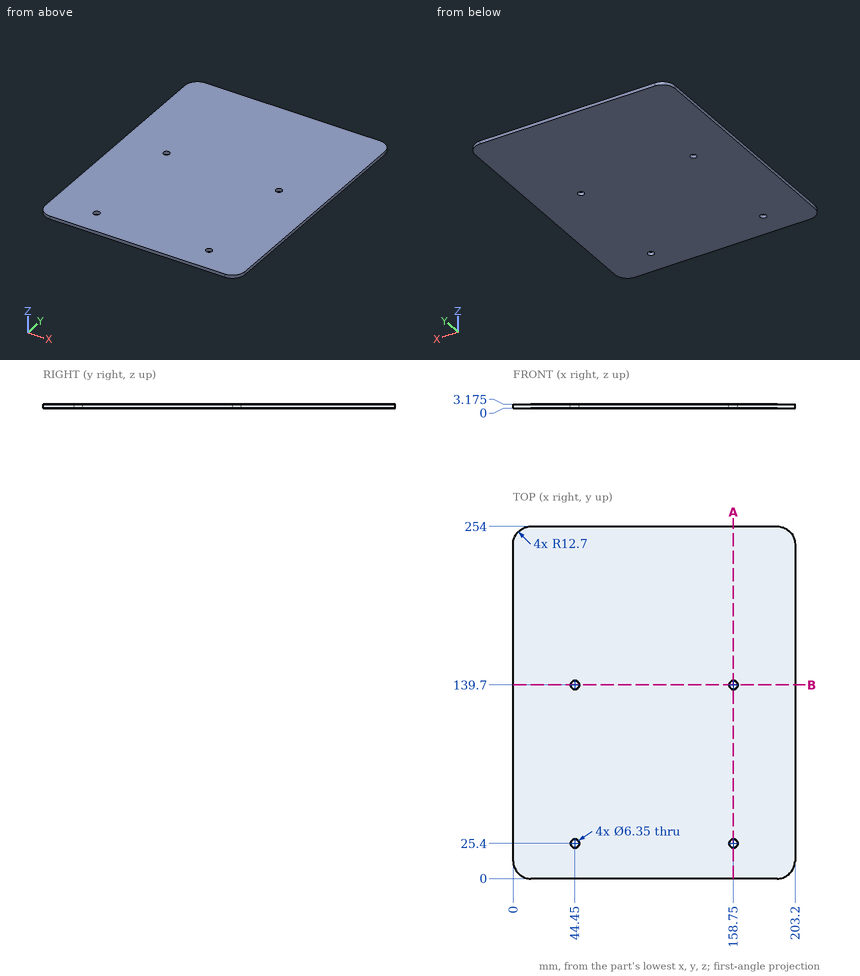
Could you check a few things on this drawing? It's one solid part, dimensions in mm from its lowest x, y, z. Round coordinates to 2 decimals unless told otherwise and drop trailing zeros. Loops run counter-clockwise (first coordinate to the right, second up) from the corner with the lowest first, then second, coordinate; pieces in that order, holes last. Notation, with made-up numbers: M 25,89.5 L 48,89.5 A10 ccw 48,99.5 Z; hole C -18.75,-16 d3. An arc over 180 degrees is marked long. Write each question's results on one line, items separated by ' | '. Start each with the question number.
(1) I want a section at B-B (y = 139.7). Please give me the cut outline in (x, z) (3 decimals), then the cut area to 3 significant figures.
(2) I want a section at A-A (x = 158.75). Please give me the cut outline in (y, z) (3 decimals).
(3) Will this pin go through, and if not, where does the flat tip stop? P1, Ø5.5, axis at x = 158.75, y = 25.4, coming from the +Z side.
(4) If I drill on probe 1 along X at (y, z) = (25.4, 0.7) (3 decimals); probe 2 along Y at (x, z) = (44.45, 2.15) (3 decimals); probe 3 along Y at (x, z) = (158, 2.35), over which ranges is the centre line in solid material (lowest first)? Write a range as from..to.
Solved:
1) outline: M 0,0 L 41.275,0 L 41.275,3.175 L 0,3.175 Z; M 47.625,0 L 155.575,0 L 155.575,3.175 L 47.625,3.175 Z; M 161.925,0 L 203.2,0 L 203.2,3.175 L 161.925,3.175 Z | area: 605 mm²
2) outline: M 0,0 L 22.225,0 L 22.225,3.175 L 0,3.175 Z; M 28.575,0 L 136.525,0 L 136.525,3.175 L 28.575,3.175 Z; M 142.875,0 L 254,0 L 254,3.175 L 142.875,3.175 Z
3) P1: passes through
4) probe 1: x = 0..41.275, 47.625..155.575, 161.925..203.2 | probe 2: y = 0..22.225, 28.575..136.525, 142.875..254 | probe 3: y = 0..22.31, 28.49..136.61, 142.79..254
